The listing builds one solid part. Answer for the finished solid, in the listing's coordinates (mm). A direction names the side the tool comes from. Give positions to 0.01 mm unless a question says otherwise; leave off trailing zeros. Answer as CSV lines item,"result". Start each with the question number.
1) For a pull along Y with two mould halves and no side action, classify faces 1 (the face through (-0.54, -2.44, 5.42)), 2 (the face through (-6.29, -4.084, 5.423)), 3 (the face through (3, 4, 11)) as pulls with the +Y half, pulls with the -Y half, needs draft (parallel to the pull), parting line crosses it, or undercut.
2) Flat-ended cylindrical pins translate along their axes: pin 1 (1.5 mm diameter, centred on x = 5, z = 2, fed in from -Y); pin 2 (1 mm diameter, centred on x = 15, z = 1.5, fed in from +Y); pin 3 (2 mm diameter, centred on y = 10, z = 3.5, fed in from +X). Find the tip coordinate at first contact, or state that the pin passes through.
3) A cutting plane is placed at A-A (z = 4.5). Give the number of separate pieces and of enclosed holes in the cut face, and give its area (3 significant figures).
4) For faces 4 (the face through (12.93, 6.41, 5.42)), 5 (the face through (4.02, 6.35, 5.58)), determine the directions among +Z, -Z, +X, -X, +Y, -Y from which every point of the face is accessible in a straight line to the end or side of a thin tool.
5) Find the intervals of material crossed by line 1 along Y through (x, z) = (11.75, 3.25); line 2 along Y through (x, z) = (-0.75, 8); line 3 along X through (y, z) = (5, 9.5), in increasing order.
```python
from build123d import *

# Parameters (mm, degrees)
SKETCH2_R           = 2.5
BOSS_EXTRUDE1_DEPTH = 11
SKETCH3_R           = 1.75
CUT_EXTRUDE1_DEPTH  = 30.961226777


with BuildPart() as part:
    # Sketch2 → Boss-Extrude1 (new body)
    with BuildSketch(Plane.XY):
        with BuildLine():
            Line((19.64777021, 14.82081493), (20.13151796, 14.038683694))
            Line((20.13151796, 14.038683694), (3.122043563, 3.518332904))
            Line((3.122043563, 3.518332904), (4.542290919, 1.222053861))
            Line((4.542290919, 1.222053861), (21.551765317, 11.74240465))
            Line((21.551765317, 11.74240465), (22.035513067, 10.960273414))
            add(Edge.make_bspline(
                [(3.945113039, -6.378564346), (11.703739539, 3.65165423), (22.035513067, 10.960273414)],
                knots=[0, 0, 0, 1, 1, 1], degree=2))
            ThreePointArc((3.945113039, -6.378564346), (-6.378571406, -3.945142993), (-3.945150053, 6.378541452))
            add(Edge.make_bspline(
                [(-3.945150053, 6.378541452), (8.494257916, 8.84079636), (19.64777021, 14.82081493)],
                knots=[0, 0, 0, 1, 1, 1], degree=2))
        make_face()
        with Locations((-1.8507e-05, -1.1447e-05)):
            Circle(SKETCH2_R, mode=Mode.SUBTRACT)
    extrude(amount=BOSS_EXTRUDE1_DEPTH)

    # Sketch3 → Cut-Extrude1 (cut, through all)
    with BuildSketch(Plane(origin=(3.945131546, -6.378552899, 0), x_dir=(0, 0, -1), z_dir=(0.5260175394579771, -0.8504737198659202, 0))):
        with Locations(Location((-5.5, 20.50592082, 0), (0, 0, 90))):
            Circle(SKETCH3_R)
        with Locations(Location((-5.5, 8.50592082, 0), (0, 0, 90))):
            Circle(SKETCH3_R)
    extrude(amount=-CUT_EXTRUDE1_DEPTH, mode=Mode.SUBTRACT)


solid = part.part
```
Ans:
1,face 1,"undercut"
1,face 2,"parting line crosses it"
1,face 3,"needs draft"
2,pin 1,"y = -5.99"
2,pin 2,"y = 12.74"
2,pin 3,"x = 22.04"
3,separate pieces,"5"
3,enclosed holes,"1"
3,area,"196 mm2"
4,face 4,"+Z, -Z"
4,face 5,"none"
5,line 1,"2.39 to 5.68, 8.85 to 11.09"
5,line 2,"-7.46 to -2.38, 2.38 to 7.07"
5,line 3,"-5.59 to 5.52, 10.65 to 14.54"
